Geometry: see drawing. Coordinates: mm, zero at the bounding-box minimum. Give positions to 0.01 mm unless a question says otherwise; leave off trailing zeros. Order: outer loops, then holes, each group sorted by start corner. A loop starts at its lowest first (then second) coordinate and runs counter-clockwise, first axis right, second up. Notation, with made-up numbers: M 50.25,-7 L 101.25,-7 A21 cw 101.25,-2 Z; hole C 0,4.25 d11. An arc over 180 degrees is marked long. Use a Markdown table: item, result.
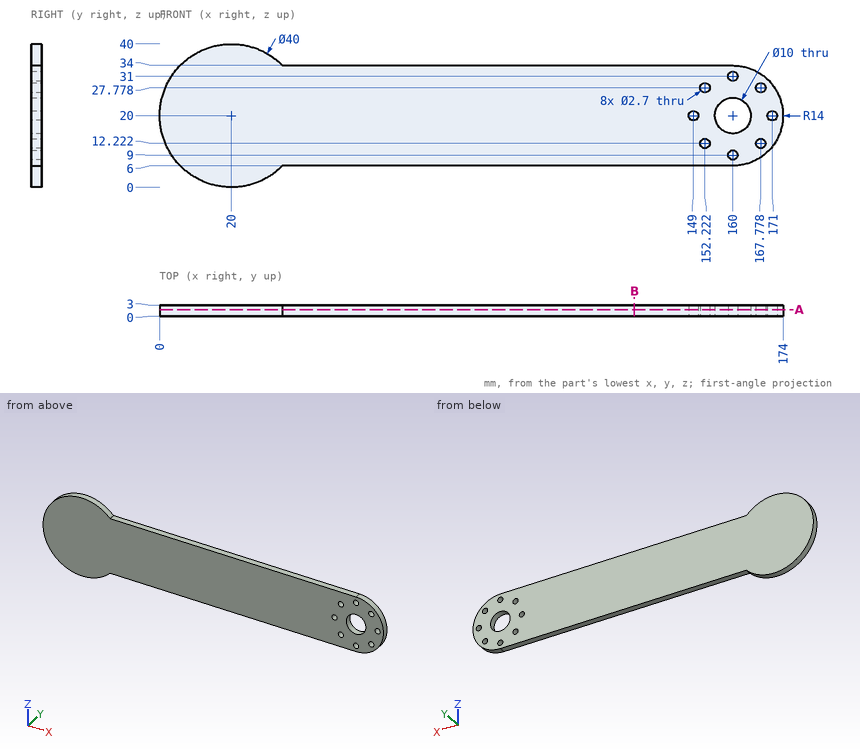
1) Cut plane A-A on y = 1.8. State how many separate pieces and enclosed holes the cut face has, and give its area (3 significant figures).
Response values:
| item | result |
|---|---|
| separate pieces | 1 |
| enclosed holes | 9 |
| area | 4,850 mm² |
2) First-contact query: pin 1 Ø1.5 at (y, z) = (1, 23) entering from -X; pin 2 Ø1 at (x, y) = (103.5, 2.5) entering from +Z. Flat tips, straight axial feed; report the tip coordinate or a pass-through.
Response values:
| item | result |
|---|---|
| pin 1 | stops at x = 0.13 |
| pin 2 | stops at z = 34 |
3) Cut plane B-B on x = 132.5. Return loops of the section in (y, z), and give its area (3 significant figures).
Response values:
| item | result |
|---|---|
| outline | M 0,6 L 3,6 L 3,34 L 0,34 Z |
| area | 84.0 mm² |
4) Material intervals for line 1 (X direction, y = 2.25, z = 20); line 2 (Z direction, x = 160, y = 1.35); line 3 (X direction, y = 0.85, z = 27) (1 decimal), sorted ascending. Write a range as from..to.
Response values:
| item | result |
|---|---|
| line 1 | x = 0..147.65, 150.35..155, 165..169.65, 172.35..174 |
| line 2 | z = 6..7.65, 10.35..15, 25..29.65, 32.35..34 |
| line 3 | x = 1.3..151.1, 153.3..166.7, 168.9..172.1 |
